Part model, mm, in its own coordinate system. Face numbers are marked on the shaded views. A direction names the side the tool comes from. Give positions to 0.01 mm unless a question says otherwise; leave off trailing zeros. Order: outer loops, then holes, each group sorted by start corner. A loop starts at its lowest first (then second) coordinate and runs counter-clockwise, first axis right, second up. Notation, with made-up numbers: M 66.5,42 L 92.5,42 A8 ccw 92.5,52 Z; hole C -10.5,-5.75 d7. An arc over 180 degrees is marked long. Return JSON: item names as keys, results as strings.
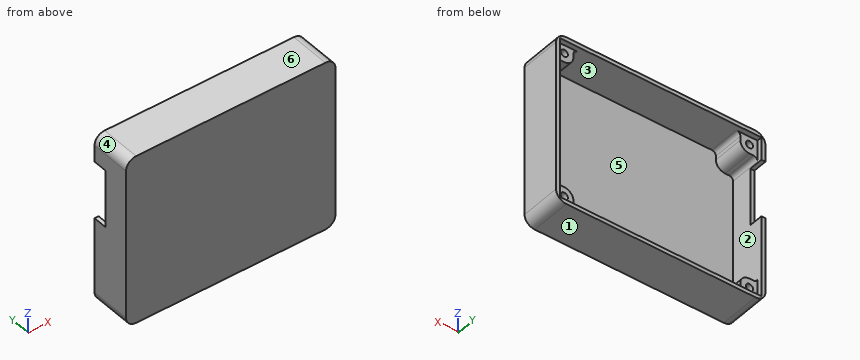
from build123d import *

# Parameters (mm, degrees)
SKETCH5_W             = 65.786
SKETCH5_H             = 53.34
BOSS_EXTRUDE1_DEPTH   = 12.7
CUT_EXTRUDE1_DEPTH    = 11.43
FILLET1_R             = 3.175
SKETCH8_W             = 63.246
SKETCH8_H             = 50.8
CUT_EXTRUDE2_DEPTH    = 1.5621
SKETCH9_W             = 15.301638829
SKETCH9_H             = 18.07026672
CUT_EXTRUDE3_DEPTH    = 4.445
BODY_MOVE_COPY1_ANGLE = 180


with BuildPart() as part:
    # Sketch5 → Boss-Extrude1 (new body)
    with BuildSketch(Plane(origin=(0, 0, 0), x_dir=(1, 0, 0), z_dir=(0, 1, 0))):
        with Locations((-7.078072202, 8.960606498)):
            Rectangle(SKETCH5_W, SKETCH5_H)
    extrude(amount=BOSS_EXTRUDE1_DEPTH)

    # Sketch7 → Cut-Extrude1 (cut)
    with BuildSketch(Plane.XZ):
        with BuildLine():
            Line((-32.033572202, -34.360606498), (17.877427798, -34.360606498))
            ThreePointArc((17.877427798, -34.360606498), (18.77545341, -33.98863211), (19.147427798, -33.090606498))
            Line((19.147427798, -33.090606498), (19.147427798, -31.820606498))
            ThreePointArc((19.147427798, -31.820606498), (19.984370171, -29.800048871), (22.004927798, -28.963106498))
            Line((22.004927798, -28.963106498), (23.274927798, -28.963106498))
            ThreePointArc((23.274927798, -28.963106498), (24.17295341, -28.59113211), (24.544927798, -27.693106498))
            Line((24.544927798, -27.693106498), (24.544927798, 9.771893502))
            ThreePointArc((24.544927798, 9.771893502), (24.17295341, 10.669919114), (23.274927798, 11.041893502))
            Line((23.274927798, 11.041893502), (22.004927798, 11.041893502))
            ThreePointArc((22.004927798, 11.041893502), (19.984370171, 11.878835875), (19.147427798, 13.899393502))
            Line((19.147427798, 13.899393502), (19.147427798, 15.169393502))
            ThreePointArc((19.147427798, 15.169393502), (18.77545341, 16.067419114), (17.877427798, 16.439393502))
            Line((17.877427798, 16.439393502), (-32.033572202, 16.439393502))
            ThreePointArc((-32.033572202, 16.439393502), (-32.931597814, 16.067419114), (-33.303572202, 15.169393502))
            Line((-33.303572202, 15.169393502), (-33.303572202, 13.899393502))
            ThreePointArc((-33.303572202, 13.899393502), (-34.140514575, 11.878835875), (-36.161072202, 11.041893502))
            Line((-36.161072202, 11.041893502), (-37.431072202, 11.041893502))
            ThreePointArc((-37.431072202, 11.041893502), (-38.329097814, 10.669919114), (-38.701072202, 9.771893502))
            Line((-38.701072202, 9.771893502), (-38.701072202, -27.693106498))
            ThreePointArc((-38.701072202, -27.693106498), (-38.329097814, -28.59113211), (-37.431072202, -28.963106498))
            Line((-37.431072202, -28.963106498), (-36.161072202, -28.963106498))
            ThreePointArc((-36.161072202, -28.963106498), (-34.140514575, -29.800048871), (-33.303572202, -31.820606498))
            Line((-33.303572202, -31.820606498), (-33.303572202, -33.090606498))
            ThreePointArc((-33.303572202, -33.090606498), (-32.931597814, -33.98863211), (-32.033572202, -34.360606498))
        make_face()
    extrude(amount=-CUT_EXTRUDE1_DEPTH, mode=Mode.SUBTRACT)

    # Fillet1
    fillet1_edges = [part.edges().sort_by_distance(p)[0] for p in [
        (-39.971072202, 6.35, 17.709393502),
        (-39.971072202, 6.35, -35.630606498),
        (25.814927798, 6.35, -35.630606498),
        (25.814927798, 6.35, 17.709393502),
    ]]
    fillet(fillet1_edges, radius=FILLET1_R)

    # Sketch8 → Cut-Extrude2 (cut)
    with BuildSketch(Plane(origin=(0, 0, 0), x_dir=(1, 0, 0), z_dir=(0, 1, 0))):
        with Locations((-7.078072202, 8.960606498)):
            Rectangle(SKETCH8_W, SKETCH8_H)
    extrude(amount=CUT_EXTRUDE2_DEPTH, mode=Mode.SUBTRACT)

    # Sketch9 → Cut-Extrude3 (cut)
    with BuildSketch(Plane(origin=(0, 0, 0), x_dir=(1, 0, 0), z_dir=(0, 1, 0))):
        with Locations((26.561690875, -0.292260142)):
            Rectangle(SKETCH9_W, SKETCH9_H)
    extrude(amount=CUT_EXTRUDE3_DEPTH, mode=Mode.SUBTRACT)

    # Sketch10 → Tap Drill for #4-40 Tap1 (revolve, cut)
    with BuildSketch(Plane(origin=(-36.161072202, 0, 13.899393502), x_dir=(0, 0, -1), z_dir=(1, 0, 0))):
        Polygon((0, 0), (0, 9.569152758), (1.1303, 8.89), (1.1303, 0), align=None)
    tap_drill_for_4_40_tap1 = revolve(axis=Axis((-36.161072202, -6.35, 13.899393502), (0, 1, 0)), mode=Mode.SUBTRACT)

    # Mirror1: Tap Drill for #4-40 Tap1 across plane
    add(tap_drill_for_4_40_tap1.mirror(Plane(origin=(-7.078072202, 0, 0), x_dir=(0, 0, 1), z_dir=(1, 0, 0))), mode=Mode.SUBTRACT)

    # Mirror2: Tap Drill for #4-40 Tap1 across plane
    add(tap_drill_for_4_40_tap1.mirror(Plane.XY.offset(-8.960606498)), mode=Mode.SUBTRACT)

    # Mirror2 copy 1 sketch → Mirror2 copy 1 (revolve, cut)
    with BuildSketch(Plane(origin=(22.004927798, 0, -31.820606498), x_dir=(0, 0, 1), z_dir=(-1, 0, 0))):
        Polygon((0, 0), (0, 9.569152758), (1.1303, 8.89), (1.1303, 0), align=None)
    revolve(axis=Axis((22.004927798, -6.35, -31.820606498), (0, 1, 0)), mode=Mode.SUBTRACT)


with BuildPart() as part_1:
    # Body-Move/Copy1: moved
    add(part.part.rotate(Axis((-7.078072202, 6.35, 0), (0, 0, 1)), BODY_MOVE_COPY1_ANGLE))


solid = part_1.part
Q1. Band-saw the part on C-C (x = -28). Give the cut face in (y, z).
Established:
{"outline": "M 0,-35.63 L 12.7,-35.63 L 12.7,-34.36 L 1.27,-34.36 L 1.27,16.44 L 12.7,16.44 L 12.7,17.71 L 0,17.71 Z"}
Q2. Probe line 1 along Z through (x, y) = (-10.5, 2.5); line 2 along X through (y, z) = (8.25, -26); line 3 along X through (y, z) = (7.5, -31). List the from-to ranges inside material, lowest first.
Established:
{"line 1": "z = -35.63 to -34.36, 16.44 to 17.71", "line 2": "x = -39.97 to -38.7, 24.54 to 25.81", "line 3": "x = -39.97 to -36.94, -35.38 to -33.42, 19.27 to 21.23, 22.78 to 25.81"}
Q3. Band-saw the part on B-B (z = -24). Give the cut face in (x, y), then the cut area to 3 significant figures.
Established:
{"outline": "M -39.97,0 L 25.81,0 L 25.81,12.7 L 24.54,12.7 L 24.54,1.27 L -38.7,1.27 L -38.7,12.7 L -39.97,12.7 Z", "area": "113 mm²"}
Q4. Band-saw the part on D-D (y = 6.5). Give the number of separate pieces and of enclosed holes in the cut face, then the cut area to 3 significant figures.
Established:
{"separate pieces": "1", "enclosed holes": "5", "area": "384 mm²"}
Q5. 3-axis set-ups, long thin cutter, end or side, ignore diameter. For the marked faces 1 and 2: which of +Z, -Z, +X, -X, +Y, -Y reach the whole face in a straight line?
Established:
{"face 1": "-Z, +X, -X, +Y, -Y", "face 2": "+Y"}
Q6. Pin check, flat tips, straight feed: pin 1 (0.6 mm diameter, centred on x = -37, y = 7, fed in from +Z); pin 2 (1.8 mm diameter, centred on x = -36.16, z = -31.82, fed in from +Y); pin 3 (3.5 mm diameter, centred on x = 20.5, z = 13, fed in from +Y); pin 4 (2 mm diameter, centred on x = -9, z = -18.5, fed in from +Y). Stop position of each tip, or through.
Established:
{"pin 1": "stops at z = 17.71", "pin 2": "stops at y = 3.67", "pin 3": "stops at y = 11.14", "pin 4": "stops at y = 1.27"}
Q7. Two-plate mould, pull along X, no slides. Class the marked faces 3, 4, 5 and 6: +X half, -X half, draft (parallel to the pull), parting line (faces both ways), or undercut.
Established:
{"face 3": "undercut", "face 4": "-X half", "face 5": "undercut", "face 6": "draft"}
